Source: CAD feature listing. Evaluate the final solid. Frame: model axes, mm. A direction names the side the tool comes from. Give positions to 0.01 mm unless a question says otherwise; leave off trailing zeros. Loops run counter-clockwise (first coordinate to the right, second up) from the corner with the lowest first, then second, coordinate; pieces in that order, holes last. Notation, with made-up numbers: (34.25, 11) -> (45.25, 11) arc R15 cw to (45.25, 18) -> close; hole circle Ø7 at (8.25, 79.5). An arc over 180 degrees is marked (long way). Return JSON: item names as keys, results as strings. Group by question number.
(1) Pin query (flat end, axial travel): pin 1 (2 mm diameter, centred on x = 0.5, y = 31, fed in from -Z); pin 2 (1.5 mm diameter, centred on y = 59, z = -1.5, fed in from -X); pin 3 (6 mm diameter, centred on x = -4.5, y = 102.5, fed in from -Z). Return the tip coordinate at first contact, or that it passes through.
(2) Cut plane B-B on y = 41.5. Return loops of the section in (x, z), then the cut area to 3 significant figures.
(3) Cut plane A-A on x = 0. Return loops of the section in (y, z).
(4) Draft query along Y for faces 1 (the face through (0.1, 143.6, -3)), 2 (the face through (0, 150, 0)), 3 (the face through (-6.93, 57.19, 2.87)). Return one class per face: released by +Y, released by -Y, zero draft, split by the parting line, or undercut.
(5) Access query for faces 4 (the face through (0, 0, 0)), 5 (the face through (1.301, 132.762, 5.857)). Directions: +Z, -Z, +X, -X, +Y, -Y. A direction counts if a zero-diameter tool reaches every point of the face in a straight line with its end or side. Return the directions, or none.
(6) Cut plane C-C on y = 127. Return loops of the section in (x, z).
(7) Ray query, line 1 (Y direction, x = -5, z = 5.5); line 2 (Y direction, x = 1.75, z = -3.75); line 3 (Y direction, x = -1.5, z = -3.5). Return the intervals inside material, ascending. Write a range as from..to.
```python
from build123d import *

# Parameters (mm, degrees)
F4_R     = 4
F5_DEPTH = 12.5


with BuildPart() as f1:
    # F0 (on Top) → F1 (revolve)
    with BuildSketch(Plane.XY):
        Polygon((-7.5, 0), (0, 0), (0, 150), (-6, 150), (-6, 116), (-7.5, 116), align=None)
    revolve(axis=Axis((0, 75, 0), (0, -1, 0)))

    # F2 (on Top) → F3 (revolve, cut)
    with BuildSketch(Plane.XY):
        Polygon((4.365895, 20), (9.365895, 16), (9.365895, 20), align=None)
    revolve(axis=Axis((12.081508, 20, 0), (1, 0, 0)), mode=Mode.SUBTRACT)

    # F4 (on Right) → F5 (cut, symmetric)
    with BuildSketch(Plane.YZ):
        with Locations((143.5, -7)):
            Circle(F4_R)
    extrude(amount=F5_DEPTH, both=True, mode=Mode.SUBTRACT)


solid = f1.part
```
Answers:
{
 "1": {"pin 1": "z = -7.5", "pin 2": "x = -7.46", "pin 3": "z = -7.35"},
 "2": {"outline": "circle Ø15 at (0, 0)", "area": "177 mm²"},
 "3": {"outline": "(0, -7.5) -> (116, -7.5) -> (116, -6) -> (139.63, -6) arc R4 cw to (147.37, -6) -> (150, -6) -> (150, 6) -> (116, 6) -> (116, 7.5) -> (0, 7.5) -> close"},
 "4": {"face 1": "undercut", "face 2": "released by +Y", "face 3": "zero draft"},
 "5": {"face 4": "+Z, -Z, +X, -X, -Y", "face 5": "+Y"},
 "6": {"outline": "circle Ø12 at (0, 0)"},
 "7": {"line 1": "0..116", "line 2": "0..141.17, 145.83..150", "line 3": "0..141.56, 145.44..150"}
}
